Geometry check sheet. Reference: the model listing, model coordinates, mm. A direction names the side the tool comes from. Coordinates: 2 decimals unless noted, no trailing zeros. Loops run counter-clockwise (first coordinate to the right, second up) from the corner with the lowest first, then second, coordinate; pieces in that order, holes last.
from build123d import *

# Parameters (mm, degrees)
SKETCH1_R               = 2.4892
BOSS_EXTRUDE1_DEPTH     = 6.35
BOSS_EXTRUDE2_START     = -6.35
BOSS_EXTRUDE2_DEPTH     = 19.05
BOSS_EXTRUDE2_START_2   = -6.555460136
BOSS_EXTRUDE2_2_DEPTH   = 19.460920272
BOSS_EXTRUDE2_START_3   = -10
BOSS_EXTRUDE2_3_DEPTH   = 3.65
CUT_EXTRUDE1_DEPTH      = 27.910448217
CUT_EXTRUDE1_DEPTH_BACK = 27.910448217
SKETCH3_W               = 2.179354936
SKETCH3_H               = 6.35


with BuildPart() as part:
    # Sketch1 → Boss-Extrude1 (new body)
    with BuildSketch(Plane(origin=(0, 0, 0), x_dir=(1, 0, 0), z_dir=(0, 1, 0))):
        with BuildLine():
            Line((9.525, -17.889269346), (-0.578271622, -16.817120786))
            Line((-0.578271622, -16.817120786), (-6.35, 0))
            Line((-6.35, 0), (12.7, 0))
            Line((12.7, 0), (12.7, -6.35))
            ThreePointArc((12.7, -6.35), (15.186560179, -13.240601753), (9.525, -17.889269346))
        make_face()
        with Locations(Location((9.525, -11.43, 0), (0, 0, 270))):
            Circle(SKETCH1_R, mode=Mode.SUBTRACT)
    extrude(amount=BOSS_EXTRUDE1_DEPTH)

    # Boss-Extrude2: read off the stored shape, not the designer's step
    # Boss-Extrude2 outline → Boss-Extrude2 (add)
    with BuildSketch(Plane.YZ.offset(BOSS_EXTRUDE2_START)):
        with BuildLine():
            ThreePointArc((11.551615481, -6.35), (12.905510296, -4.996105185), (11.551615481, -3.642210371))
            Line((11.551615481, -3.642210371), (6.35, 0))
            Line((6.35, 0), (0, 0))
            Line((0, 0), (-5.201615481, -3.642210371))
            ThreePointArc((-5.201615481, -3.642210371), (-6.555510296, -4.996105185), (-5.201615481, -6.35))
            Line((-5.201615481, -6.35), (11.551615481, -6.35))
        make_face()
    extrude(amount=BOSS_EXTRUDE2_DEPTH)

    # Boss-Extrude2 2 outline → Boss-Extrude2 2 (add)
    with BuildSketch(Plane(origin=(0, 0, 0), x_dir=(1, 0, 0), z_dir=(0, 1, 0)).offset(BOSS_EXTRUDE2_START_2)):
        Polygon((-8.529354936, 6.35), (-6.35, 0), (-6.35, 6.35), align=None)
    extrude(amount=BOSS_EXTRUDE2_2_DEPTH)

    # Boss-Extrude2 3 outline → Boss-Extrude2 3 (cut)
    with BuildSketch(Plane.YZ.offset(BOSS_EXTRUDE2_START_3)):
        with BuildLine():
            Line((12.905460136, 0), (6.35, 0))
            Line((6.35, 0), (11.551615481, -3.642210371))
            ThreePointArc((11.551615481, -3.642210371), (12.504834401, -4.034645431), (12.905460136, -4.984450993))
            Line((12.905460136, -4.984450993), (12.905460136, 0))
        make_face()
        with BuildLine():
            ThreePointArc((12.905460136, -5.007759378), (12.504834401, -5.95756494), (11.551615481, -6.35))
            Line((11.551615481, -6.35), (12.905460136, -6.35))
            Line((12.905460136, -6.35), (12.905460136, -5.007759378))
        make_face()
        with BuildLine():
            Line((0, 0), (-6.555460136, 0))
            Line((-6.555460136, 0), (-6.555460136, -4.984450993))
            ThreePointArc((-6.555460136, -4.984450993), (-6.154834401, -4.034645431), (-5.201615481, -3.642210371))
            Line((-5.201615481, -3.642210371), (0, 0))
        make_face()
        with BuildLine():
            ThreePointArc((-5.201615481, -6.35), (-6.154834401, -5.95756494), (-6.555460136, -5.007759378))
            Line((-6.555460136, -5.007759378), (-6.555460136, -6.35))
            Line((-6.555460136, -6.35), (-5.201615481, -6.35))
        make_face()
    extrude(amount=BOSS_EXTRUDE2_3_DEPTH, mode=Mode.SUBTRACT)

    # Sketch3 → Cut-Extrude1 (cut, two sides: drawn at the far end of the back side and taken through both)
    with BuildSketch(Plane.XZ.offset(-CUT_EXTRUDE1_DEPTH_BACK)):
        with Locations((-7.439677468, -3.175)):
            Rectangle(SKETCH3_W, SKETCH3_H)
    extrude(amount=CUT_EXTRUDE1_DEPTH + CUT_EXTRUDE1_DEPTH_BACK, mode=Mode.SUBTRACT)


solid = part.part
(1) Sectioned sample at A-A on y = 5.25. Record the cut outline in (x, z) (3 decimals), and give its area (3 significant figures).
Findings:
outline: (-6.35, -6.35) - (12.7, -6.35) - (12.7, 6.35) arc R6.35 ccw to (9.525, 17.889) - (-0.578, 16.817) - (-6.35, 0) - close; hole circle Ø4.978 at (9.525, 11.43)
area: 401 mm2
(2) Draft check along Z on faces 5 (the flat face through (3.042, 8.914, -1.796)), 6 (the cylindrical face through (3.042, 12.905, -5.026)), 7 (the cylindrical face through (11.993, 3.131, 11.106)). Enter one of: +Z half, -Z half, draft (parallel to the pull), parting line (faces both ways), or undercut.
Findings:
face 5: +Z half
face 6: parting line
face 7: undercut
(3) Scan lines: L1, parallel to Y at x = -2.75, z = 3.75; L2, parallel to Z at x = 10.5, y = 2. Record each from-to range of solid material in increasing order.
Findings:
L1: y = 0 to 6.35
L2: z = -6.35 to 9.14, 13.72 to 17.74
(4) Sectioned sample at D-D on x = 8.75. Record the cut outline in (y, z), and give its area (3 significant figures).
Findings:
outline: (-5.2, -6.35) - (11.55, -6.35) arc R1.35 ccw to (11.55, -3.64) - (6.35, 0) - (6.35, 9.06) - (0, 9.06) - (0, 0) - (-5.2, -3.64) arc R1.35 ccw to start; (0, 13.8) - (6.35, 13.8) - (6.35, 17.81) - (0, 17.81) - close
area: 176 mm2
(5) Sectioned sample at C-C on x = 4.25. Record the cut outline in (y, z).
Findings:
outline: (-5.2, -6.35) - (11.55, -6.35) arc R1.35 ccw to (11.55, -3.64) - (6.35, 0) - (6.35, 17.33) - (0, 17.33) - (0, 0) - (-5.2, -3.64) arc R1.35 ccw to start
(6) Access from +Z, -Z, +X, -X, +Y, -Y to the whole of each face (thin tool, end or side, straight path). Record for faces 1 (the flat face through (5, 0, 9)), 2 (the flat face through (12.7, 3, -1)), 3 (the flat face through (4.54, 3.13, 17.36)), 4 (the flat face through (5, 6.35, 9)).
Findings:
face 1: +Z, +X, -X, -Y
face 2: -Z, +X, +Y, -Y
face 3: +Z, -X, +Y, -Y
face 4: +Z, +X, -X, +Y
(7) Gauge pin test, flat ends, axial feed: pin 1 Ø1.5 at (y, z) = (3.5, 12.5) entering from +X; pin 2 Ø12 at (x, z) = (-2.5, 5.5) entering from +Y; pin 3 Ø5.5 at (x, z) = (2, 8) entering from -Y. Record the tip position at first contact, or that the pin passes through.
Findings:
pin 1: stops at x = 15.41
pin 2: stops at y = 7.06
pin 3: stops at y = 0
(8) Sectioned sample at B-B on z = 13.5. Record the cut outline in (x, y).
Findings:
outline: (-1.72, 0) - (8.14, 0) - (8.14, 6.35) - (-1.72, 6.35) - close; (10.91, 0) - (15.11, 0) - (15.11, 6.35) - (10.91, 6.35) - close
